from build123d import *

# Parameters (mm, degrees)
SKETCH_1_W               = 20
SKETCH_1_H               = 18
EXTRUDE_1_DEPTH          = 20
SKETCH_2_W               = 16
SKETCH_2_H               = 14
CUT_EXTRUDE_1_DEPTH      = 18
CUT_EXTRUDE_2_DEPTH      = 28.49545417
CUT_EXTRUDE_2_DEPTH_BACK = 28.49545417
CUT_EXTRUDE_3_DEPTH      = 23.472205054
CUT_EXTRUDE_3_DEPTH_BACK = 23.472205054
SKETCH_5_R               = 2.75
CUT_EXTRUDE_4_DEPTH      = 28.147743921
CUT_EXTRUDE_4_DEPTH_BACK = 28.147743921
SKETCH_6_R               = 2.75


with BuildPart() as part:
    # 스케치1 → 보스-돌출1 (new body)
    with BuildSketch(Plane.XY):
        Rectangle(SKETCH_1_W, SKETCH_1_H)
    extrude(amount=EXTRUDE_1_DEPTH)

    # 스케치2 → 컷-돌출1 (cut)
    with BuildSketch(Plane.XY.offset(20)):
        with Locations((2, 0)):
            Rectangle(SKETCH_2_W, SKETCH_2_H)
    extrude(amount=-CUT_EXTRUDE_1_DEPTH, mode=Mode.SUBTRACT)

    # 스케치4 → 컷-돌출2 (cut, two sides: drawn at the far end of the back side and taken through both)
    with BuildSketch(Plane(origin=(0, -7, 0), x_dir=(1, 0, 0), z_dir=(0, 1, 0)).offset(-CUT_EXTRUDE_2_DEPTH_BACK)):
        Polygon((-6, -20), (10, -2), (10, -20), align=None)
    extrude(amount=CUT_EXTRUDE_2_DEPTH + CUT_EXTRUDE_2_DEPTH_BACK, mode=Mode.SUBTRACT)

    # 스케치5 → 컷-돌출3 (cut, two sides: drawn at the far end of the back side and taken through both)
    with BuildSketch(Plane.XY.offset(2).offset(-CUT_EXTRUDE_3_DEPTH_BACK)):
        Circle(SKETCH_5_R)
    extrude(amount=CUT_EXTRUDE_3_DEPTH + CUT_EXTRUDE_3_DEPTH_BACK, mode=Mode.SUBTRACT)

    # 스케치6 → 컷-돌출4 (cut, two sides: drawn at the far end of the back side and taken through both)
    with BuildSketch(Plane(origin=(-6, 0, 0), x_dir=(0, 0, -1), z_dir=(1, 0, 0)).offset(-CUT_EXTRUDE_4_DEPTH_BACK)):
        with Locations(Location((-12, 0, 0), (0, 0, 90))):
            Circle(SKETCH_6_R)
    extrude(amount=CUT_EXTRUDE_4_DEPTH + CUT_EXTRUDE_4_DEPTH_BACK, mode=Mode.SUBTRACT)


solid = part.part
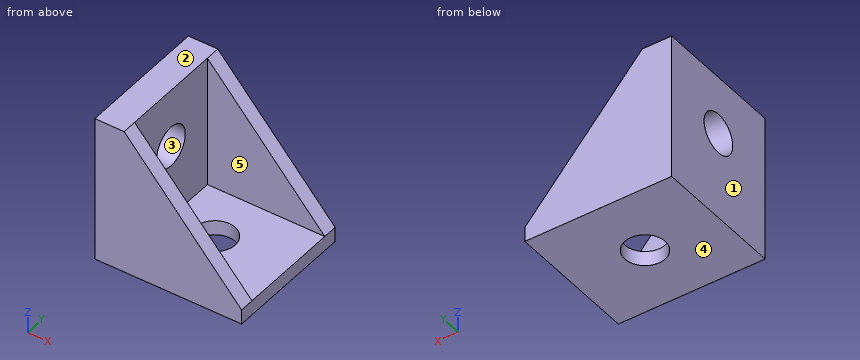
Could you check a few things on this model? Use its own coordinates, in mm. Face numbers are marked on the shaded views. A direction names the side the tool comes from. Give positions to 0.01 mm unless a question says otherwise; leave off trailing zeros. Loops run counter-clockwise (first coordinate to the right, second up) from the corner with the lowest first, then second, coordinate; pieces in that order, holes last. Notation, with made-up numbers: M 32,-31.75 L 87,-31.75 A37 ccw 87,4.25 Z; hole C 69,14 d9. An arc over 180 degrees is marked long. Answer as a JSON object with one key per item and string values.
Q1. Suppose I cut it at B-B, the plane y = 0. List the corners of the cut face in (x, z) for me.
Values found:
{"outline": "M -10,0 L -2.75,0 L -2.75,2 L -6,2 L -6,9.25 L -10,9.25 Z; M -10,14.75 L -6,14.75 L -6,20 L -10,20 Z; M 2.75,0 L 10,0 L 10,2 L 2.75,2 Z"}
Q2. Suppose I cut it at C-C, the plane x = -7. List the corners of the cut face in (y, z) for me.
Values found:
{"outline": "M -9,0 L 9,0 L 9,20 L -9,20 Z; hole C 0,12 d5.5"}
Q3. Suppose I cut it at D-D, the plane z = 9.75. List the corners of the cut face in (x, y) for me, plus the area to 3 significant figures.
Values found:
{"outline": "M -10,-9 L 3.11,-9 L 3.11,-7 L -6,-7 L -6,-1.58 L -10,-1.58 Z; M -10,1.58 L -6,1.58 L -6,7 L 3.11,7 L 3.11,9 L -10,9 Z", "area": "95.8 mm²"}
Q4. If we mould it in two halves opening along Z, with no side actions, what happens to the marked faces 1, 2 and 3? For each: pulls with the +Z half, pulls with the -Z half, needs draft (parallel to the pull), parting line crosses it, or undercut.
Values found:
{"face 1": "needs draft", "face 2": "pulls with the +Z half", "face 3": "undercut"}
Q5. If I drill on probe 1 along Y at (x, z) = (0, 0.6); probe 2 along X at (y, z) = (0, 1.05); probe 3 along Y at (x, z) = (-5.5, 15.25), over which ranges is the centre line in solid material (lowest first)? Write a range as [from, to].
Values found:
{"probe 1": "y = [-9, -2.75], [2.75, 9]", "probe 2": "x = [-10, -2.75], [2.75, 10]", "probe 3": "y = [-9, -7], [7, 9]"}
Q6. For the marked faces 4 and 5, which set-ups out of +Z, -Z, +X, -X, +Y, -Y let a thin tool reach every point of the face, with its end or its side?
Values found:
{"face 4": "-Z, +X, -X, +Y, -Y", "face 5": "+Z, +X"}
Q7. For P1, Ø8, axis at x = -1.5, y = 0.5, coming from the +Z side; P2, Ø6, axis at y = 5.5, z = 16.5, coming from the +X side; P3, Ø10, axis at y = 7, z = 5, coming from the +X side; P4, Ø4, axis at y = 2, z = 13.5, coming from the +X side, each with a flat end and sliding along its axis, tell me the tip position at first contact or that it passes through.
Values found:
{"P1": "stops at z = 2", "P2": "stops at x = -0.58", "P3": "stops at x = 10", "P4": "stops at x = -6"}
Q8. Suppose I cut it at A-A, the plane x = 0. List the corners of the cut face in (y, z) for me, plus the area to 3 significant figures.
Values found:
{"outline": "M -9,0 L -2.75,0 L -2.75,2 L -7,2 L -7,13.25 L -9,13.25 Z; M 2.75,0 L 9,0 L 9,13.25 L 7,13.25 L 7,2 L 2.75,2 Z", "area": "70.0 mm²"}
